Autodesk Inventor part; units mm, degrees
ref_plane "YZ Plane" through (0, 0, 0) normal (1, 0, 0) x (0, 1, 0)
ref_plane "XZ Plane" through (0, 0, 0) normal (0, 1, 0) x (-1, 0, 0)
ref_plane "XY Plane" through (0, 0, 0) normal (0, 0, 1) x (1, 0, 0)
sketch "Sketch1" plane through (0, 0, 0) normal (0, 1, 0) x (-1, 0, 0)
  line L0 (55, 48.2) -> (-10.0469, 48.2)
  line L1 (55, -48.2) -> (55, 48.2)
  line L2 (55, 48.2) -> (-55, -48.2) construction
  line L3 (-55, 48.2) -> (55, -48.2) construction
  arc A0 (-10.0469, 48.2) -> (-10.0469, -48.2) centre (425.3935, 0) ccw
  line L4 (-12.7065, -11.1355) -> (-12.7065, 11.1355)
  line L5 (55, -48.2) -> (-10.0469, -48.2)
  point P0 (0, 0)
  dimension "d82" = 876.2
  dimension "d83" = 425.3935
  dimension "d85" = 96.4
  dimension "d86" = 48.2
  dimension "d87" = 55
  dimension "d88" = 67.7065
extrude "Extrusion1" add sketch "Sketch1" along normal blind 10
sketch "Sketch2" plane through (0, 10, 0) normal (0, 1, 0) x (1, 0, 0)
  circle A0 centre (40, 43.2) radius 2
  circle A1 centre (0, 43.2) radius 2
  circle A2 centre (-40, 43.2) radius 2
  line L0 (55, -48.2) -> (55, 48.2)
  line L1 (-55, 48.2) -> (-55, -48.2)
  line L2 (55, 48.2) -> (-55, 48.2)
  circle A3 centre (40, -43.2) radius 2
  circle A4 centre (-22.4766, -43.2) radius 2
  circle A5 centre (-40, -43.2) radius 2
  line L3 (-55, -48.2) -> (10.0469, -48.2)
  point P0 (0, 0)
  point P1 (-22.4766, -48.2)
  dimension "d4" = 15
  dimension "d5" = 15
  dimension "d6" = 4
  dimension "d7" = 4
  dimension "d8" = 4
  dimension "d9" = 5
  dimension "d10" = 5
  dimension "d11" = 5
  dimension "d12" = 4
  dimension "d13" = 4
  dimension "d14" = 4
  dimension "d15" = 5
  dimension "d16" = 5
  dimension "d17" = 5
  dimension "d25" = 15
  dimension "d26" = 15
hole "Hole1" at (40, 10, -43.2) at (0, 10, -43.2) at (-40, 10, -43.2) at (-40, 10, 43.2) at (-22.4766, 10, 43.2) at (40, 10, 43.2) direction (0, -1, 0) diameter 3 end through all
sketch "Sketch5" plane through (0, 0, 0) normal (0, -1, 0) x (1, 0, 0)
  point P0 (0, 0)
sketch "Sketch6" plane through (-55, 0, -48.2) normal (-1, 0, 0) x (0, 0, 1)
  line L0 (96.4, 0) -> (96.4, 10)
  line L1 (96.4, 0) -> (0, 0)
  line L2 (96.4, 10) -> (0, 10)
  line L3 (0, 10) -> (0, 0)
  line L4 (0, 0) -> (96.4, 0)
  line L5 (96.4, 0) -> (96.4, 10)
  point P0 (48.2, 0)
extrude "Extrusion4" add sketch "Sketch6" along normal blind 10
sketch "Sketch7" plane through (0, 10, 0) normal (0, 1, 0) x (1, 0, 0)
  line L0 (0, -7.5) -> (-50, -7.5)
  line L1 (-50, -7.5) -> (-50, 7.5)
  line L2 (-50, 7.5) -> (0, 7.5)
  line L3 (0, 7.5) -> (0, -7.5)
  line L4 (0, -7.5) -> (-50, 7.5) construction
  line L5 (-50, -7.5) -> (0, 7.5) construction
  line L6 (-65, -48.2) -> (-65, 48.2)
  point P0 (0, 0)
  point P1 (-25, 0)
  dimension "d66" = 15
  dimension "d67" = 50
  dimension "d68" = 15
  dimension "d89" = 7.5
extrude "Extrusion5" cut sketch "Sketch7" against normal blind 10
sketch "Sketch8" plane through (0, 10, 0) normal (0, 1, 0) x (1, 0, 0)
  line L0 (-50, -7.5) -> (-50, 7.5)
  line L1 (-50, 7.5) -> (0, 7.5)
  line L2 (0, 7.5) -> (0, 17.5)
  line L3 (0, 17.5) -> (-50, 17.5)
  line L4 (-50, 17.5) -> (-50, 7.5)
  line L5 (0, -7.5) -> (-50, -7.5)
  line L6 (-50, -7.5) -> (0, -7.5)
  line L7 (0, -7.5) -> (0, -17.5)
  line L8 (0, -17.5) -> (-50, -17.5)
  line L9 (-50, -17.5) -> (-50, -7.5)
  point P0 (0, 0)
  point P1 (0, -7.5)
  dimension "d71" = 10
  dimension "d72" = 10
extrude "Extrusion6" add sketch "Sketch8" along normal blind 10
sketch "Sketch9" plane through (-50, 10, 17.5) normal (0, 0, 1) x (1, 0, 0)
  circle A0 centre (10, 5) radius 2.5
  circle A1 centre (40, 5) radius 2.5
  line L0 (0, 0) -> (0, 10)
  line L1 (50, 0) -> (50, 10)
  line L2 (0, 10) -> (50, 10)
  point P0 (50, -10)
  point P1 (0, 5)
  dimension "d75" = 5
  dimension "d77" = 10
  dimension "d79" = 5
  dimension "d105" = 40
  dimension "d106" = 5
  dimension "d107" = 5
extrude "Extrusion7" cut sketch "Sketch9" against normal through all
sketch "Sketch10" plane through (0, 10, 0) normal (0, 1, 0) x (1, 0, 0)
  line L0 (-65, -48.2) -> (10.0469, -48.2)
  arc A0 (10.0469, -48.2) -> (10.0469, 48.2) centre (-425.3935, 0) ccw
  line L1 (-65, -48.2) -> (14.2881, -48.2)
  line L2 (14.2881, -48.2) -> (14.2881, -21.9629)
  line L3 (-65, -17.5) -> (-65, -48.2)
  line L4 (10.0469, 48.2) -> (-65, 48.2)
  line L5 (-65, 48.2) -> (14.2881, 48.2)
  line L6 (14.2881, 48.2) -> (14.2881, 20.8403)
  line L7 (-65, 17.5) -> (-65, 48.2)
  line L8 (0, -48.2) -> (14.2881, -48.2)
  line L9 (14.2881, -48.2) -> (14.2881, 48.2)
  line L10 (14.2881, 48.2) -> (0, 48.2)
  line L11 (0, 17.5) -> (0, -17.5)
  line L12 (0, -17.5) -> (-65, -17.5)
  line L13 (0, 17.5) -> (-65, 17.5)
  line L14 (-50, -7.5) -> (-50, 7.5)
  point P0 (0, 0)
  point P1 (-50, 0)
  dimension "d90" = 35
  dimension "d91" = 65
  dimension "d92" = 17.5
extrude "Extrusion8" cut sketch "Sketch10" against normal blind 10 contours L3 L12 L11 L13 L7 L4 A0 L0
sketch "Sketch11" plane through (-65, 0, -48.2) normal (-1, 0, 0) x (0, 0, 1)
  line L0 (65.7, 10) -> (55.7, 10)
  line L1 (30.7, 0) -> (65.7, 0)
  line L2 (65.7, 0) -> (65.7, 10)
  line L3 (65.7, 10) -> (30.7, 10)
  line L4 (30.7, 10) -> (30.7, 0)
  point P0 (48.2, 0)
extrude "Extrusion9" add sketch "Sketch11" along normal blind 15
sketch "Sketch12" plane through (0, 20, 0) normal (0, 1, 0) x (1, 0, 0)
  line L0 (0, 17.5) -> (-50, 17.5)
  line L1 (0, -17.5) -> (-80, -17.5)
  line L2 (0, 17.5) -> (-5, 17.5)
  line L3 (-5, 17.5) -> (-5, -17.5)
  line L4 (-5, -17.5) -> (0, -17.5)
  line L5 (0, -17.5) -> (0, 17.5)
  point P0 (0, 0)
  dimension "d97" = 5
extrude "Extrusion10" add sketch "Sketch12" along normal blind 5
fillet "Fillet1" radius 5 2 edges at (-5, 20, -12.5) (-5, 20, 12.5)
sketch "Sketch13" plane through (-50, 10, 17.5) normal (0, 0, 1) x (1, 0, 0)
  circle A0 centre (40, 5) radius 2.5
  circle A1 centre (10, 5) radius 2.5
  line L0 (50, 15) -> (50, -10)
  line L1 (45, 15) -> (50, 15)
  arc A2 (40, 10) -> (45, 15) centre (40, 15) ccw
  line L2 (0, 10) -> (40, 10)
  line L3 (0, 0) -> (0, 10)
  line L4 (-30, 0) -> (0, 0)
  line L5 (-30, -10) -> (-30, 0)
  line L6 (50, -10) -> (-30, -10)
  point P0 (50, -10)
extrude "Extrusion11" add sketch "Sketch13" along normal blind 0.2
sketch "Sketch14" plane through (-50, 10, -17.5) normal (0, 0, -1) x (-1, 0, 0)
  arc A0 (-45, 17.9) -> (-50, -48.1) centre (388.1, -48.1) ccw
  line L0 (0, 0) -> (30, 0)
  line L1 (-50, 15) -> (-50, -10)
  line L2 (-50, 15) -> (-50, -48.1)
  line L3 (-50, 15) -> (-45, 17.9)
  point P0 (-50, -10)
  dimension "d108" = 876.2
  dimension "d109" = 48.1
  dimension "d110" = 438.1
extrude "Extrusion12" cut sketch "Sketch14" against normal through all
sketch "Sketch15" plane through (-50, 10, -17.5) normal (0, 0, -1) x (-1, 0, 0)
  line L0 (-40, 10) -> (0, 10)
  line L1 (-40, 10) -> (-53.6921, 10)
  arc A0 (-45, 15) -> (-40, 10) centre (-40, 15) ccw
  line L2 (-53.6921, 10) -> (-41.0966, 19.8783)
  line L3 (-41.0966, 19.8783) -> (-40, 10)
  point P0 (-50, -10)
extrude "Extrusion13" cut sketch "Sketch15" against normal through all
sketch "Sketch16" plane through (0, 20, 0) normal (0, 1, 0) x (1, 0, 0)
  line L0 (-3.8696, -7.5) -> (-3.8696, -17.7)
  line L1 (-50, -17.7) -> (-50, -7.5)
  line L2 (-50, -12.6) -> (-50, -7.5)
  line L3 (-3.8696, -7.5) -> (-50, -7.5)
  line L4 (-50, -7.5) -> (0.7476, -7.5)
  line L5 (0.7476, -7.5) -> (0.7476, -12.6)
  line L6 (0.7476, -12.6) -> (-50, -12.6)
  point P0 (0, 0)
  point P1 (-3.8696, -12.6)
extrude "Extrusion14" cut sketch "Sketch16" against normal through all
sketch "Sketch17" plane through (-50, 10, 17.7) normal (0, 0, 1) x (1, 0, 0)
  line L0 (-30, 0) -> (-30, -10)
  line L1 (-30, -9.8) -> (48.9645, -9.8)
  line L2 (48.9645, -9.8) -> (48.9645, -10.6043)
  line L3 (48.9645, -10.6043) -> (-30, -10.6043)
  line L4 (-30, -10.6043) -> (-30, -9.8)
  line L5 (-30, -10) -> (48.3401, -10)
  point P0 (50, -10)
  dimension "d117" = 0.2
extrude "Extrusion15" cut sketch "Sketch17" against normal blind 25.2
properties part number "ReleaseMec2.0SideMec"
Source: CAD feature listing. Evaluate the final solid. Frame: model axes, mm. A direction names the side the tool comes from. Coordinates: 2 decimals unless noted, no trailing zeros. Loops run counter-clockwise (first coordinate to the right, second up) from the corner with the lowest first, then second, coordinate; pieces in that order, holes last. Notation, with made-up numbers: M -24.75,56 L 29.25,56 A31 cw 29.25,92 Z; hole C 41,78 d7. An arc over 180 degrees is marked long. Use a Markdown table: item, result. Add a question column.
Q1. Access query for faces 1 (the flat face through (-50, 5, 3)), 2 (the flat face through (-50, 15, 15)), 3 (the cylindrical face through (-37.69, 14.04, -12.43)), 4 (the flat face through (-59, 0.2, 8)). Directions: +Z, -Z, +X, -X, +Y, -Y. A direction counts if a zero-diameter tool reaches every point of the face in a straight line with its end or side. Return the directions, or none.
Q2. Draft query along X for faces 5 (the cylindrical face through (-37.69, 15.96, 15.11)), 6 (the flat face through (-26, 10, 12.6)), 7 (the flat face through (-50, 15, -13)). Return one class per face: pulls with the +X half, pulls with the -X half, needs draft (parallel to the pull), parting line crosses it, or undercut.
Q3. Material intervals for L1, parallel to Y at x = -10, z = -13.75; L2, parallel to Y at x = -40, z = 15.5; L3, parallel to Z at x = -38.5, y = 1.5, sorted ascending.
Q4. Section query D-D, the plane x = -51.5. Return loops of the section in (y, z), and give its area (3 significant figures).
Q5. Section query B-B, the plane x = -40. Return loops of the section in (y, z).
Q6. Section query A-A, the plane z = 15. Return loops of the section in (x, y), and give its area (3 significant figures).
Q7. First-contact query: pin 1 (4 mm diameter, centred on x = -40, y = 15, fed in from -Z); pin 2 (3 mm diameter, centred on y = 12.5, z = -13.5, fed in from -X); pin 3 (3 mm diameter, centred on y = 3, z = 0, fed in from +X); pin 4 (3 mm diameter, centred on x = -72, z = -7, fed in from +Y). Flat tips, straight axial feed; report the tip coordinate or a pass-through.
Q8. Section query C-C, the plane y = 13.5. Return loops of the section in (x, z), and give its area (3 significant figures).
Result:
| question | item | result |
|---|---|---|
| 1 | face 1 | +X, +Y, -Y |
| 1 | face 2 | +Z, -Z, -X, +Y |
| 1 | face 3 | +Z, -Z |
| 1 | face 4 | +Z, +X, -X, -Y |
| 2 | face 5 | undercut |
| 2 | face 6 | needs draft |
| 2 | face 7 | pulls with the -X half |
| 3 | L1 | y = 0 to 12.5, 17.5 to 20 |
| 3 | L2 | y = 0.2 to 12.5, 17.5 to 20 |
| 3 | L3 | z = -17.5 to -7.5, 12.6 to 17.7 |
| 4 | outline | M 0,-17.5 L 10,-17.5 L 10,17.7 L 0.2,17.7 L 0.2,-7.5 L 0,-7.5 Z |
| 4 | area | 347 mm2 |
| 5 | outline | M 0,-17.5 L 12.5,-17.5 L 12.5,-7.5 L 0,-7.5 Z; M 0.2,12.6 L 12.5,12.6 L 12.5,17.7 L 0.2,17.7 Z; M 17.5,-17.5 L 20,-17.5 L 20,-7.5 L 17.5,-7.5 Z; M 17.5,12.6 L 20,12.6 L 20,17.7 L 17.5,17.7 Z |
| 6 | outline | M -80,0.2 L -1.68,0.2 A438.1 ccw -3.87,20 L -50,20 L -50,10 L -80,10 Z; hole C -40,15 d5; hole C -10,15 d5 |
| 6 | area | 1,190 mm2 |
| 7 | pin 1 | passes through |
| 7 | pin 2 | stops at x = -50 |
| 7 | pin 3 | stops at x = -50 |
| 7 | pin 4 | stops at y = 10 |
| 8 | outline | M -50,-17.5 L -42,-17.5 L -42,-7.5 L -50,-7.5 Z; M -50,12.6 L -42,12.6 L -42,17.7 L -50,17.7 Z; M -38,-17.5 L -12,-17.5 L -12,-7.5 L -38,-7.5 Z; M -38,12.6 L -12,12.6 L -12,17.7 L -38,17.7 Z; M -8,-17.5 L -3.05,-17.5 L -3.05,-7.5 L -8,-7.5 Z; M -8,12.6 L -3.05,12.6 L -3.05,17.7 L -8,17.7 Z |
| 8 | area | 588 mm2 |
